Can you work these out from the model? Positions are in its coordinate system, mm. A direction names the side the tool comes from. Round coordinates to 2 decimals unless told otherwise and drop trailing zeros. Loops run counter-clockwise (first coordinate to the right, second up) from the corner with the lowest first, then second, coordinate; pieces in that order, holes last. Notation, with made-up numbers: M 6,19.5 L 40,19.5 A6 ccw 40,28.5 Z; hole C 22,59.25 d8. An arc over 180 degrees is marked long. Answer as CSV lines item,"result".
from build123d import *

# Parameters (mm, degrees)
F1_DEPTH = 5
F2_R     = 25
F3_R     = 20
F3_R_2   = 12.5
F4_DEPTH = 15


with BuildPart() as f1:
    # F0 (on Front) → F1 (new body)
    with BuildSketch(Plane.XZ):
        with BuildLine():
            Line((15, 0), (15, 27.12932))
            ThreePointArc((15, 27.12932), (0, 31), (-15, 27.12932))
            Line((-15, 27.12932), (-15, 0))
            Line((-15, 0), (0, 0))
            Line((0, 0), (15, 0))
        make_face()
        with BuildLine():
            ThreePointArc((-15, 27.12932), (-15.748016, -26.70206), (31, 0))
            ThreePointArc((31, 0), (26.70206, 15.748016), (15, 27.12932))
            Line((15, 27.12932), (15, 0))
            Line((15, 0), (0, 0))
            Line((0, 0), (-15, 0))
            Line((-15, 0), (-15, 27.12932))
        make_face()
        with BuildLine():
            ThreePointArc((-15, 27.12932), (0, 31), (15, 27.12932))
            Line((15, 27.12932), (15, 50))
            Line((15, 50), (-15, 50))
            Line((-15, 50), (-15, 27.12932))
        make_face()
    extrude(amount=F1_DEPTH)

    # F2
    f2_edges = [f1.edges().sort_by_distance(p)[0] for p in [
        (-15, -2.5, 27.12932),
        (15, -2.5, 27.12932),
    ]]
    fillet(f2_edges, radius=F2_R)

    # F3 (on face) → F4 (join)
    with BuildSketch(Plane.XZ.offset(5)):
        Circle(F3_R)
        Circle(F3_R_2, mode=Mode.SUBTRACT)
    extrude(amount=F4_DEPTH)


solid = f1.part
Item 1: On a 3-axis mill with a long thin cutter (end or side, diameter ignored), from which of +Z, -Z, +X, -X, +Y, -Y can I reach the whole of each face in a straight line? I mean faces 1 (the face through (6.5, -5, 19.1)), 2 (the face through (15, -2, 45)), 3 (the face through (0, -2, 50)). Say none if no direction works.
Output:
face 1,"-Y"
face 2,"+Z, +X, +Y, -Y"
face 3,"+Z, +X, -X, +Y, -Y"
Item 2: We'd pull the mould along X, two halves only. Please class faces 4 (the face through (16.906, -2.535, 29.617)), 5 (the face through (-15, -2, 45)), 6 (the face through (0, -5, 0)): released by +X, released by -X, zero draft, split by the parting line, or undercut.
Output:
face 4,"released by +X"
face 5,"released by -X"
face 6,"undercut"
Item 3: If I drill on line 1 along Z through (x, y) = (0, -13.5); line 2 along Y through (x, z) = (-15, -21); line 3 along X through (y, z) = (-9.25, -5.5), over which ranges is the centre line in solid material (lowest first)? Write a range as from..to.
Output:
line 1,"z = -20..-12.5, 12.5..20"
line 2,"y = -5..0"
line 3,"x = -19.23..-11.22, 11.22..19.23"
Item 4: If we section it at C-C on y = -4: Write out the boundary of the cut face in (x, z).
Output:
outline,"M -22.14,21.7 A31 ccw long 31,0 A31 ccw 22.14,21.7 A25 cw 15,39.19 L 15,50 L -15,50 L -15,39.19 A25 cw Z"
Item 5: If we section it at A-A on x = 0: Write out the boundary of the cut face in (y, z).
Output:
outline,"M -20,-20 L -5,-20 L -5,-31 L 0,-31 L 0,50 L -5,50 L -5,20 L -20,20 L -20,12.5 L -5,12.5 L -5,-12.5 L -20,-12.5 Z"
Item 6: If we section it at D-D on y = -10.5: Write out the boundary of the cut face in (x, z).
Output:
outline,"C 0,0 d40; hole C 0,0 d25"
Item 7: If we section it at B-B on z = 3: Write out the boundary of the cut face in (x, y), then the cut area to 3 significant figures.
Output:
outline,"M -30.85,-5 L -19.77,-5 L -19.77,-20 L -12.13,-20 L -12.13,-5 L 12.13,-5 L 12.13,-20 L 19.77,-20 L 19.77,-5 L 30.85,-5 L 30.85,0 L -30.85,0 Z"
area,"538 mm2"
Item 8: Will these pins go through, and if not, where does the flat tip stop? pin 1 (4 mm diameter, centred on y = -2.5, z = 45, fed in from -X); pin 2 (1.5 mm diameter, centred on y = -2.5, z = 45, fed in from +X); pin 3 (1 mm diameter, centred on x = 21.5, z = 1, fed in from +Y); pin 4 (1.5 mm diameter, centred on x = -20, y = -4, fed in from -Z).
Output:
pin 1,"stops at x = -15"
pin 2,"stops at x = 15"
pin 3,"stops at y = 0"
pin 4,"stops at z = -24.3"
